Part model, mm, in its own coordinate system. Coordinates: 2 decimals unless noted, no trailing zeros. Order: outer loops, then holes, each group sorted by start corner. A loop starts at its lowest first (then second) coordinate and runs counter-clockwise, first axis right, second up. Notation, with made-up numbers: (29, 62.5) - (76, 62.5) arc R8 ccw to (76, 70.5) - close; hole circle Ø5 at (57.5, 72.25). An arc over 180 degrees is marked (long way). Use a Markdown table: item, result. Add a question column.
1) Two-plate mould, pull along X, no slides. Class faces 1 (the face through (0, 28, 1)), 2 (the face through (-14.091, -24.196, 0.986)), 3 (the face through (1.13, -24.27, 0.99)), 4 (the face through (24.196, -14.091, 0.986)): +X half, -X half, draft (parallel to the pull), parting line (faces both ways), or undercut.
2) Saw through at B-B on y = 0. List the corners of the cut face in (x, z).
3) Saw through at C-C on x = 6.5. List the corners of the cut face in (y, z), then the cut area to 3 significant figures.
4) Saw through at A-A on z = 0.7. List the corners of the cut face in (x, y), then the cut area to 3 significant figures.
5) Wall check: L1, parallel to Y at x = 0, z = 0.7; L2, parallel to Y at x = -19.5, z = 0.5; L3, parallel to Y at x = -3.5, z = 0.1. Give the ranges that are in metal, low to high. Write a range as [from, to].
6) Drop a flat-ended pin along its axis: P1, Ø2.5, axis at x = 0, y = 22.5, coming from the +Z side. Give the stop position or say it passes through.
7) Saw through at D-D on y = 11.25. List the corners of the cut face in (x, z).
Autodesk Fusion 360 part; units mm, degrees
sketch "Sketch1" plane through (0, 0, 0) normal (0, 0, 1) x (1, 0, 0)
  line L0 (-7.5026, 28) -> (-20.4974, 20.4974)
  line L1 (-20.4974, 20.4974) -> (-28, 7.5026)
  line L2 (-28, 7.5026) -> (-28, -7.5026)
  line L3 (-28, -7.5026) -> (-20.4974, -20.4974)
  line L4 (-20.4974, -20.4974) -> (-7.5026, -28)
  line L5 (-7.5026, -28) -> (7.5026, -28)
  line L6 (7.5026, -28) -> (20.4974, -20.4974)
  line L7 (20.4974, -20.4974) -> (28, -7.5026)
  line L8 (28, -7.5026) -> (28, 7.5026)
  line L9 (28, 7.5026) -> (20.4974, 20.4974)
  line L10 (20.4974, 20.4974) -> (7.5026, 28)
  line L11 (7.5026, 28) -> (-7.5026, 28)
  circle A0 centre (0, 0) radius 22.5 construction
  line L12 (0, 0) -> (0, 28) construction
  circle A1 centre (0, 22.5) radius 2.1
  circle A2 centre (-19.4856, 11.25) radius 2.1
  circle A3 centre (-19.4856, -11.25) radius 2.1
  circle A4 centre (0, -22.5) radius 2.1
  circle A5 centre (19.4856, -11.25) radius 2.1
  circle A6 centre (19.4856, 11.25) radius 2.1
  circle A7 centre (0, 0) radius 15
  dimension "d1" = 28
  dimension "d2" = 45
  dimension "d3" = 4.2
  dimension "d5" = 360
  dimension "d6" = 30
extrude "Extrude1" add sketch "Sketch1" along normal blind 2
Results are:
| question | item | result |
|---|---|---|
| 1 | face 1 | draft |
| 1 | face 2 | -X half |
| 1 | face 3 | undercut |
| 1 | face 4 | +X half |
| 2 | outline | (-28, 0) - (-15, 0) - (-15, 2) - (-28, 2) - close; (15, 0) - (28, 0) - (28, 2) - (15, 2) - close |
| 3 | outline | (-28, 0) - (-13.52, 0) - (-13.52, 2) - (-28, 2) - close; (13.52, 0) - (28, 0) - (28, 2) - (13.52, 2) - close |
| 3 | area | 57.9 mm2 |
| 4 | outline | (-28, -7.5) - (-20.5, -20.5) - (-7.5, -28) - (7.5, -28) - (20.5, -20.5) - (28, -7.5) - (28, 7.5) - (20.5, 20.5) - (7.5, 28) - (-7.5, 28) - (-20.5, 20.5) - (-28, 7.5) - close; hole circle Ø4.2 at (-19.49, -11.25); hole circle Ø4.2 at (-19.49, 11.25); hole circle Ø30 at (0, 0); hole circle Ø4.2 at (0, -22.5); hole circle Ø4.2 at (0, 22.5); hole circle Ø4.2 at (19.49, -11.25); hole circle Ø4.2 at (19.49, 11.25) |
| 4 | area | 1,730 mm2 |
| 5 | L1 | [-28, -24.6], [-20.4, -15], [15, 20.4], [24.6, 28] |
| 5 | L2 | [-21.07, -13.35], [-9.15, 9.15], [13.35, 21.07] |
| 5 | L3 | [-28, -14.59], [14.59, 28] |
| 6 | P1 | through |
| 7 | outline | (-25.84, 0) - (-21.59, 0) - (-21.59, 2) - (-25.84, 2) - close; (-17.39, 0) - (-9.92, 0) - (-9.92, 2) - (-17.39, 2) - close; (9.92, 0) - (17.39, 0) - (17.39, 2) - (9.92, 2) - close; (21.59, 0) - (25.84, 0) - (25.84, 2) - (21.59, 2) - close |
